from build123d import *

# Parameters (mm, degrees)
SKETCH1_W           = 62
SKETCH1_H           = 45
SKETCH1_R           = 2
BOSS_EXTRUDE1_DEPTH = 10
SKETCH2_R           = 8
CUT_EXTRUDE1_DEPTH  = 7


with BuildPart() as part:
    # Sketch1 → Boss-Extrude1 (new body)
    with BuildSketch(Plane.XY):
        Rectangle(SKETCH1_W, SKETCH1_H)
        with Locations((-15, -15)):
            Circle(SKETCH1_R, mode=Mode.SUBTRACT)
        with Locations((-15, 15)):
            Circle(SKETCH1_R, mode=Mode.SUBTRACT)
        with Locations((15, 15)):
            Circle(SKETCH1_R, mode=Mode.SUBTRACT)
        with Locations((15, -15)):
            Circle(SKETCH1_R, mode=Mode.SUBTRACT)
    extrude(amount=BOSS_EXTRUDE1_DEPTH)

    # Chamfer1
    # the kernel refuses this chamfer: 7 mm, written as the material it takes off along each edge
    with BuildSketch(Plane(origin=(-26.333333333, 17.833333333, 5.333333333), x_dir=(0, 0.7071067811865476, -0.7071067811865476), z_dir=(-0.5773502691896257, 0.5773502691896257, 0.5773502691896257)), Plane(origin=(-26.333333333, -17.833333333, 5.333333333), x_dir=(0, 0.7071067811865476, 0.7071067811865476), z_dir=(-0.5773502691896257, -0.5773502691896257, 0.5773502691896257)), Plane(origin=(26.333333333, 17.833333333, 5.333333333), x_dir=(-0.7071067811865476, 0.7071067811865476, 0), z_dir=(0.5773502691896257, 0.5773502691896257, 0.5773502691896257))) as chamfer1_piece_1:
        Polygon((-4.949747468, -2.857738033), (4.949747468, -2.857738033), (0, 5.715476066), align=None)
    extrude(amount=8.891194146, mode=Mode.SUBTRACT)
    with BuildSketch(Plane(origin=(26.333333333, -17.833333333, 5.333333333), x_dir=(0, 0.7071067811865476, 0.7071067811865476), z_dir=(0.5773502691896257, -0.5773502691896257, 0.5773502691896257))) as chamfer1_piece_2:
        Polygon((-4.949747468, 2.857738033), (4.949747468, 2.857738033), (0, -5.715476066), align=None)
    extrude(amount=8.891194146, mode=Mode.SUBTRACT)
    with BuildSketch(Plane(origin=(-31, 40.501780916, 10), x_dir=(-0.02749587661058661, 0, -0.9996219169112968), z_dir=(0, -1, 0)), Plane(origin=(31, -40.501780916, 10), x_dir=(0.02749587661058661, 0, -0.9996219169112968), z_dir=(0, 1, 0))) as chamfer1_piece_3:
        with BuildLine():
            Line((7.200712366, 0), (-0.395830084, 7.189824555))
            Line((-0.395830084, 7.189824555), (-0.535777153, 7.185975132))
            ThreePointArc((-0.535777153, 7.185975132), (-0.238904589, 3.593784808), (-0.139947068, -0.003849423))
            Line((-0.139947068, -0.003849423), (0.003849423, -0.139947068))
            ThreePointArc((0.003849423, -0.139947068), (3.601483653, -0.040989547), (7.204561789, -0.139947068))
            Line((7.204561789, -0.139947068), (7.200712366, 0))
        make_face()
    extrude(amount=81.003561832, mode=Mode.SUBTRACT)
    with BuildSketch(Plane(origin=(-49.001780916, -22.5, 10), x_dir=(0, -0.02749587661058661, -0.9996219169112968), z_dir=(1, 0, 0)), Plane(origin=(49.001780916, 22.5, 10), x_dir=(0, 0.02749587661058661, -0.9996219169112968), z_dir=(-1, 0, 0))) as chamfer1_piece_4:
        with BuildLine():
            Line((7.200712366, 0), (-0.395830084, 7.189824555))
            Line((-0.395830084, 7.189824555), (-0.535777153, 7.185975132))
            ThreePointArc((-0.535777153, 7.185975132), (-0.238904589, 3.593784808), (-0.139947068, -0.003849423))
            Line((-0.139947068, -0.003849423), (0.003849423, -0.139947068))
            ThreePointArc((0.003849423, -0.139947068), (3.601483653, -0.040989547), (7.204561789, -0.139947068))
            Line((7.204561789, -0.139947068), (7.200712366, 0))
        make_face()
    extrude(amount=98.003561832, mode=Mode.SUBTRACT)
    with BuildSketch(Plane(origin=(31, -22.5, -18.001780916), x_dir=(-0.9996219169112968, -0.027495876610586605, 0), z_dir=(0, 0, 1)), Plane(origin=(-31, 22.5, -18.001780916), x_dir=(0.9996219169112968, 0.027495876610586605, 0), z_dir=(0, 0, 1)), Plane(origin=(31, 22.5, -18.001780916), x_dir=(0.02749587661058661, -0.9996219169112968, 0), z_dir=(0, 0, 1))) as chamfer1_piece_5:
        with BuildLine():
            Line((7.200712366, 0), (-0.395830084, -7.189824555))
            Line((-0.395830084, -7.189824555), (-0.535777153, -7.185975132))
            ThreePointArc((-0.535777153, -7.185975132), (-0.238904589, -3.593784808), (-0.139947068, 0.003849423))
            Line((-0.139947068, 0.003849423), (0.003849423, 0.139947068))
            ThreePointArc((0.003849423, 0.139947068), (3.601483653, 0.040989547), (7.204561789, 0.139947068))
            Line((7.204561789, 0.139947068), (7.200712366, 0))
        make_face()
    extrude(amount=46.003561832, mode=Mode.SUBTRACT)
    with BuildSketch(Plane(origin=(-31, -22.5, -18.001780916), x_dir=(0.9996219169112968, -0.027495876610586605, 0), z_dir=(0, 0, 1))) as chamfer1_piece_6:
        with BuildLine():
            Line((7.200712366, 0), (-0.395830084, 7.189824555))
            Line((-0.395830084, 7.189824555), (-0.535777153, 7.185975132))
            ThreePointArc((-0.535777153, 7.185975132), (-0.238904589, 3.593784808), (-0.139947068, -0.003849423))
            Line((-0.139947068, -0.003849423), (0.003849423, -0.139947068))
            ThreePointArc((0.003849423, -0.139947068), (3.601483653, -0.040989547), (7.204561789, -0.139947068))
            Line((7.204561789, -0.139947068), (7.200712366, 0))
        make_face()
    extrude(amount=46.003561832, mode=Mode.SUBTRACT)

    # Sketch2 → Cut-Extrude1 (cut)
    with BuildSketch(Plane.XY.offset(10)):
        with Locations((-15, 15)):
            Circle(SKETCH2_R)
        with Locations((-15, -15)):
            Circle(SKETCH2_R)
        with Locations((15, -15)):
            Circle(SKETCH2_R)
        with Locations((15, 15)):
            Circle(SKETCH2_R)
    extrude(amount=-CUT_EXTRUDE1_DEPTH, mode=Mode.SUBTRACT)


solid = part.part
Geometry: final body of the model. Coordinates: model frame, mm. A direction names the side the tool comes from. Round coordinates to 2 decimals unless told otherwise and drop trailing zeros. Loops run counter-clockwise (first coordinate to the right, second up) from the corner with the lowest first, then second, coordinate; pieces in that order, holes last.
Q1. Section B-B on z = 2.25. Return loops of the section in (x, y), plus the area to 3 significant figures.
Q2. Section D-D on z = 7.75. Return loops of the section in (x, y).
Q3. Material intervals for L1, parallel to Y at x = 15, z = 1.6; L2, parallel to X at y = 15, z = 1; L3, parallel to X at y = 15, z = 4.75, sorted ascending.
Q4. Section A-A on x = 15. Return loops of the section in (y, z), plus the area to 3 significant figures.
Q5. Access query for faces 5 (the flat face through (-0.2, -19.8, 5.7)), 6 (the cylindrical face through (15, -7, 7)). Directions: +Z, -Z, +X, -X, +Y, -Y. A direction counts if a zero-diameter tool reaches every point of the face in a straight line with its end or side. Return the directions, or none.
Q6. Pull-direction query (X, two-part tool) for faces 1 (the cylindrical face through (-15, -7, 7)), 2 (the flat face through (-22.3, -19.8, 5.7)), 3 (the flat face through (-27.5, -19, 1.5)), 4 (the flat face through (-13, -16, 3)); classes: released by +X, released by -X, zero draft, split by the parting line, or undercut.
Q7. Section C-C on y = -14. Return loops of the section in (x, z), plus the area to 3 significant figures.
Q8. Pin query (flat end, axial travel): P1, Ø8, axis at x = -17.5, y = -14, coming from the +Z side; P2, Ø3, axis at x = 2.5, z = 5.5, coming from the -Y side; P3, Ø3, axis at x = 15, y = -15, coming from the +Z side; P4, Ø6, axis at y = 7, z = 8, coming from the +X side. Return the tip coordinate at first contact, or that it passes through.
Evaluation:
1. outline: (-31, -15.5) - (-24, -22.5) - (24, -22.5) - (31, -15.5) - (31, 15.5) - (24, 22.5) - (-24, 22.5) - (-31, 15.5) - close; hole circle Ø4 at (-15, -15); hole circle Ø4 at (-15, 15); hole circle Ø4 at (15, -15); hole circle Ø4 at (15, 15)
1. area: 2,640 mm2
2. outline: (-26.25, -15.5) - (-24, -17.75) - (-22.51, -17.75) arc R8 cw (long way) to (-7.49, -17.75) - (7.49, -17.75) arc R8 cw (long way) to (22.51, -17.75) - (24, -17.75) - (26.25, -15.5) - (26.25, 15.5) - (24, 17.75) - (22.51, 17.75) arc R8 cw (long way) to (7.49, 17.75) - (-7.49, 17.75) arc R8 cw (long way) to (-22.51, 17.75) - (-24, 17.75) - (-26.25, 15.5) - close
3. L1: y = -22.5 to -17, -13 to 13, 17 to 22.5
3. L2: x = -31 to -17, -13 to 13, 17 to 31
3. L3: x = -29.25 to -23, -7 to 7, 23 to 29.25
4. outline: (-22.5, 0) - (-17, 0) - (-17, 3) - (-22.5, 3) - close; (-13, 0) - (13, 0) - (13, 3) - (7, 3) - (7, 10) - (-7, 10) - (-7, 3) - (-13, 3) - close; (17, 0) - (22.5, 0) - (22.5, 3) - (17, 3) - close
4. area: 209 mm2
5. face 5: +Z, +X, -X, -Y
5. face 6: +Z
6. face 1: undercut
6. face 2: zero draft
6. face 3: released by -X
6. face 4: undercut
7. outline: (-31, 0) - (-16.73, 0) - (-16.73, 3) - (-22.94, 3) - (-22.94, 10) - (-24, 10) - (-31, 3) - close; (-13.27, 0) - (13.27, 0) - (13.27, 3) - (7.06, 3) - (7.06, 10) - (-7.06, 10) - (-7.06, 3) - (-13.27, 3) - close; (16.73, 0) - (31, 0) - (31, 3) - (24, 10) - (22.94, 10) - (22.94, 3) - (16.73, 3) - close
7. area: 328 mm2
8. P1: stops at z = 3
8. P2: stops at y = -21.5
8. P3: passes through
8. P4: stops at x = 29
